Input: part model. Units: mm. Frame: model coordinates. A direction names the side the tool comes from. Coordinates: 2 decimals unless noted, no trailing zeros. Write each loop counter-clockwise with the first axis right and the second up, starting at its lowest first coordinate (ties: lowest second). Pieces come first, ordered by that corner, then holes. Notation, with made-up numbers: M -16.75,23.5 L 30.25,23.5 A21 cw 30.25,31.5 Z; hole C 58.5,-14.75 d11. An arc over 180 degrees is marked long. Write each question's results on one line, items separated by ' | '. Start each with the question number.
1. Section query A-A, the plane z = 10.5. Output: boundary loops of the cut face in (x, y) (3 decimals).
2. Ray query, probe 1 along Z at (x, y) = (99.5, -15) (3 decimals); probe 2 along Y at (x, z) = (19, 7.5) (3 decimals); probe 3 along Y at (x, z) = (196.5, -21). Return the intervals inside material, ascending.
3. Section query C-C, the plane x = 143.5. Output: boundary loops of the cut face in (y, z) (3 decimals), and give its area (3 significant figures).
4. Pull-direction query (Z, two-part tool) for faces 3 (the flat face through (103, 0, -25.4)), 4 (the flat face through (103, 0, -22.225)), 5 (the flat face through (0, -3, -22.5)); classes: +Z half, -Z half, draft (parallel to the pull), parting line (faces both ways), or undercut.
5. Section query B-B, the plane y = -15. Output: boundary loops of the cut face in (x, z) (3 decimals).
6. Set-up query: faces 1 (the flat face through (103, 38.1, 0)), 2 (the flat face through (103, 0, 22.225)). Return all of +Z, -Z, +X, -X, +Y, -Y with unobstructed straight access to the full face (end or side cutting, diameter ignored); none if empty.
```python
from build123d import *

# Parameters (mm, degrees)
F0_W     = 76.2
F0_H     = 50.8
F0_W_2   = 69.85
F0_H_2   = 44.45
F2_DEPTH = 209.55
F3_R     = 3.175


# Not quite as in the source:
# - a variable given as a bare number and used for a length is read in inches; the dataset says mm whatever the document's units were


with BuildPart() as f2:
    # F0 (on Right) → F2 (new body)
    with BuildSketch(Plane.YZ):
        Rectangle(F0_W, F0_H)
        Rectangle(F0_W_2, F0_H_2, mode=Mode.SUBTRACT)
    extrude(amount=F2_DEPTH)

    # F3
    f3_edges = [f2.edges().sort_by_distance(p)[0] for p in [
        (104.775, 38.1, 25.4),
        (104.775, 38.1, -25.4),
        (104.775, -38.1, -25.4),
        (104.775, -38.1, 25.4),
        (104.775, 34.925, -22.225),
        (104.775, 34.925, 22.225),
        (104.775, -34.925, 22.225),
        (104.775, -34.925, -22.225),
    ]]
    fillet(f3_edges, radius=F3_R)


solid = f2.part
```
Answer:
1) outline: M 0,-38.1 L 209.55,-38.1 L 209.55,-34.925 L 0,-34.925 Z; M 0,34.925 L 209.55,34.925 L 209.55,38.1 L 0,38.1 Z
2) probe 1: -25.4 to -22.225, 22.225 to 25.4 | probe 2: -38.1 to -34.925, 34.925 to 38.1 | probe 3: -38.1 to -34.26, 34.26 to 38.1
3) outline: M -38.1,-22.225 A3.175 ccw -34.925,-25.4 L 34.925,-25.4 A3.175 ccw 38.1,-22.225 L 38.1,22.225 A3.175 ccw 34.925,25.4 L -34.925,25.4 A3.175 ccw -38.1,22.225 Z; hole M -34.925,-19.05 A3.175 ccw -31.75,-22.225 L 31.75,-22.225 A3.175 ccw 34.925,-19.05 L 34.925,19.05 A3.175 ccw 31.75,22.225 L -31.75,22.225 A3.175 ccw -34.925,19.05 Z | area: 766 mm^2
4) face 3: -Z half | face 4: undercut | face 5: draft
5) outline: M 0,-25.4 L 209.55,-25.4 L 209.55,-22.225 L 0,-22.225 Z; M 0,22.225 L 209.55,22.225 L 209.55,25.4 L 0,25.4 Z
6) face 1: +Z, -Z, +X, -X, +Y | face 2: +X, -X
